from build123d import *

# Parameters (mm, degrees)
F0_W     = 952.5
F0_H     = 508
F1_DEPTH = 177.8
F2_W     = 165.1
F2_H     = 139.7
F3_DEPTH = 177.801
F4_R     = 25.4


with BuildPart() as f1:
    # F0 (on Front) → F1 (new body)
    with BuildSketch(Plane.XZ):
        with Locations((476.25, 254)):
            Rectangle(F0_W, F0_H)
    extrude(amount=F1_DEPTH)

    # F2 (on face) → F3 (cut, through all)
    with BuildSketch(Plane.XZ.offset(177.8)):
        with Locations((82.55, 69.85)):
            Rectangle(F2_W, F2_H)
        with Locations((869.95, 69.85)):
            Rectangle(F2_W, F2_H)
    extrude(amount=-F3_DEPTH, mode=Mode.SUBTRACT)

    # F4
    f4_edges = [f1.edges().sort_by_distance(p)[0] for p in [
        (165.1, -88.9, 139.7),
        (787.4, -88.9, 139.7),
    ]]
    fillet(f4_edges, radius=F4_R)


solid = f1.part
Design review of the part built by this model. Coordinates are the model's own, in mm. A direction names the side the tool comes from. Coordinates: 2 decimals unless noted, no trailing zeros. Loops run counter-clockwise (first coordinate to the right, second up) from the corner with the lowest first, then second, coordinate; pieces in that order, holes last.
Item 1: Add section B-B (x = 92.5). Write out the cut boundary in (y, z), and give its area (3 significant figures).
Completed:
outline: (-177.8, 139.7) - (0, 139.7) - (0, 508) - (-177.8, 508) - close
area: 65,500 mm2
Item 2: Wall thickness on L1, parallel to X at y = -36.5, z = 67; L2, parallel to Z at x = 849.5, y = -149: over which ranges is each line inside the solid? List them lowest first.
Completed:
L1: x = 165.1 to 787.4
L2: z = 139.7 to 508
Item 3: Add section C-C (z = 54.5). Write out the cut boundary in (x, y).
Completed:
outline: (165.1, -177.8) - (787.4, -177.8) - (787.4, 0) - (165.1, 0) - close
Item 4: For faces 1 (the flat face through (0, -88, 321)), 2 (the flat face through (882, -90, 139.7)), 3 (the flat face through (69, -90, 139.7)), list the 3-axis set-ups (+Z, -Z, +X, -X, +Y, -Y) from which the entire face can be reached by the end or side of a thin tool; tool diameter is ignored.
Completed:
face 1: +Z, -Z, -X, +Y, -Y
face 2: -Z, +X, +Y, -Y
face 3: -Z, -X, +Y, -Y
Item 5: Add section A-A (y = -71.5). Write out the cut boundary in (x, z).
Completed:
outline: (0, 139.7) - (139.7, 139.7) arc R25.4 cw to (165.1, 114.3) - (165.1, 0) - (787.4, 0) - (787.4, 114.3) arc R25.4 cw to (812.8, 139.7) - (952.5, 139.7) - (952.5, 508) - (0, 508) - close
